Part model, mm, in its own coordinate system. A direction names the side the tool comes from. Round coordinates to 2 decimals unless told otherwise and drop trailing zeros. Write each loop counter-clockwise with the first axis right and the second up, starting at its lowest first coordinate (ties: lowest second). Pieces come first, ordered by that corner, then holes. Notation, with made-up numbers: (-1, -39.5) -> (15, -39.5) arc R26 ccw to (15, -23.5) -> close; hole circle Ø6 at (23.5, 31.25). An arc over 180 degrees is marked (long way). Return JSON: item names as keys, results as strings. Group by question number.
(1) Saw through at C-C (x = 20). List the corners of the cut face in (y, z), plus the area to 3 significant figures.
(2) Drop flat-ended pins along their axis: pin 1 Ø1 at (x, z) = (10, 6.5) entering from -Y; pin 2 Ø6 at (x, z) = (-7, 6) entering from -Y; pin 3 Ø1 at (y, z) = (2.5, 5) entering from -X. Give the stop position or say it passes through.
(3) Mould opens along Y. For faces 3 (the flat face through (0, 0, 9.5)), 4 (the flat face through (13, 0, 10)), 5 (the cylindrical face through (-1.53, 11.656, 10.76)) say: +Y half, -Y half, draft (parallel to the pull), parting line (faces both ways), or undercut.
(4) Tool access for faces 1 (the flat face through (0, 0, 11.5)), 2 (the cylindrical face through (-10.143, 3.194, 4.684)): list every direction of +Z, -Z, +X, -X, +Y, -Y with a clear straight run to the whole face (end or side of a thin tool).
(5) Drill centre lines: L1, parallel to Y at x = 0, z = 7.75; L2, parallel to Y at x = -1.5, z = 2.25; L3, parallel to Z at x = -9.5, y = -16.5. Where is each one in solid material? Low to high. Write a range as from..to.
(6) Saw through at A-A (x = 0). List the corners of the cut face in (y, z).
(7) Saw through at D-D (z = 7). List the corners of the cut face in (x, y).
from build123d import *

# Parameters (mm, degrees)
SKETCH1_R           = 30
BOSS_EXTRUDE1_DEPTH = 10
SKETCH2_R           = 11.755971956
BOSS_EXTRUDE3_DEPTH = 1.5
SKETCH5_R           = 2.658250205
CUT_EXTRUDE4_DEPTH  = 26
SKETCH6_R           = 10.634150048
CUT_EXTRUDE5_DEPTH  = 9.5


with BuildPart() as part:
    # Sketch1 → Boss-Extrude1 (new body)
    with BuildSketch(Plane.XY):
        Circle(SKETCH1_R)
    extrude(amount=BOSS_EXTRUDE1_DEPTH)

    # Sketch2 → Boss-Extrude3 (add, symmetric)
    with BuildSketch(Plane.XY.offset(10)):
        Circle(SKETCH2_R)
    extrude(amount=BOSS_EXTRUDE3_DEPTH, both=True)

    # Sketch5 → Cut-Extrude4 (cut)
    with BuildSketch(Plane.XY.offset(10)):
        with Locations((0, -21.20336232)):
            Circle(SKETCH5_R)
        with Locations((-21.20336232, 0)):
            Circle(SKETCH5_R)
        with Locations((0, 21.20336232)):
            Circle(SKETCH5_R)
        with Locations((21.20336232, 0)):
            Circle(SKETCH5_R)
    extrude(amount=-CUT_EXTRUDE4_DEPTH, mode=Mode.SUBTRACT)

    # Sketch6 → Cut-Extrude5 (cut)
    with BuildSketch(Plane(origin=(0, 0, 0), x_dir=(-1, 0, 0), z_dir=(0, 0, -1))):
        Circle(SKETCH6_R)
    extrude(amount=-CUT_EXTRUDE5_DEPTH, mode=Mode.SUBTRACT)


solid = part.part
Computed values:
{
 "1": {"outline": "(-22.36, 0) -> (-2.37, 0) -> (-2.37, 10) -> (-22.36, 10) -> close; (2.37, 0) -> (22.36, 0) -> (22.36, 10) -> (2.37, 10) -> close", "area": "400 mm2"},
 "2": {"pin 1": "y = -28.46", "pin 2": "y = -29.73", "pin 3": "x = -29.93"},
 "3": {"face 3": "undercut", "face 4": "draft", "face 5": "parting line"},
 "4": {"face 1": "+Z, +X, -X, +Y, -Y", "face 2": "-Z"},
 "5": {"L1": "-30..-23.86, -18.55..-10.63, 10.63..18.55, 23.86..30", "L2": "-29.96..-23.4, -19.01..-10.53, 10.53..19.01, 23.4..29.96", "L3": "0..10"},
 "6": {"outline": "(-30, 0) -> (-23.86, 0) -> (-23.86, 10) -> (-30, 10) -> close; (-18.55, 0) -> (-10.63, 0) -> (-10.63, 9.5) -> (10.63, 9.5) -> (10.63, 0) -> (18.55, 0) -> (18.55, 10) -> (11.76, 10) -> (11.76, 11.5) -> (-11.76, 11.5) -> (-11.76, 10) -> (-18.55, 10) -> close; (23.86, 0) -> (30, 0) -> (30, 10) -> (23.86, 10) -> close"},
 "7": {"outline": "circle Ø60 at (0, 0); hole circle Ø5.32 at (-21.2, 0); hole circle Ø21.27 at (0, 0); hole circle Ø5.32 at (0, -21.2); hole circle Ø5.32 at (0, 21.2); hole circle Ø5.32 at (21.2, 0)"}
}
